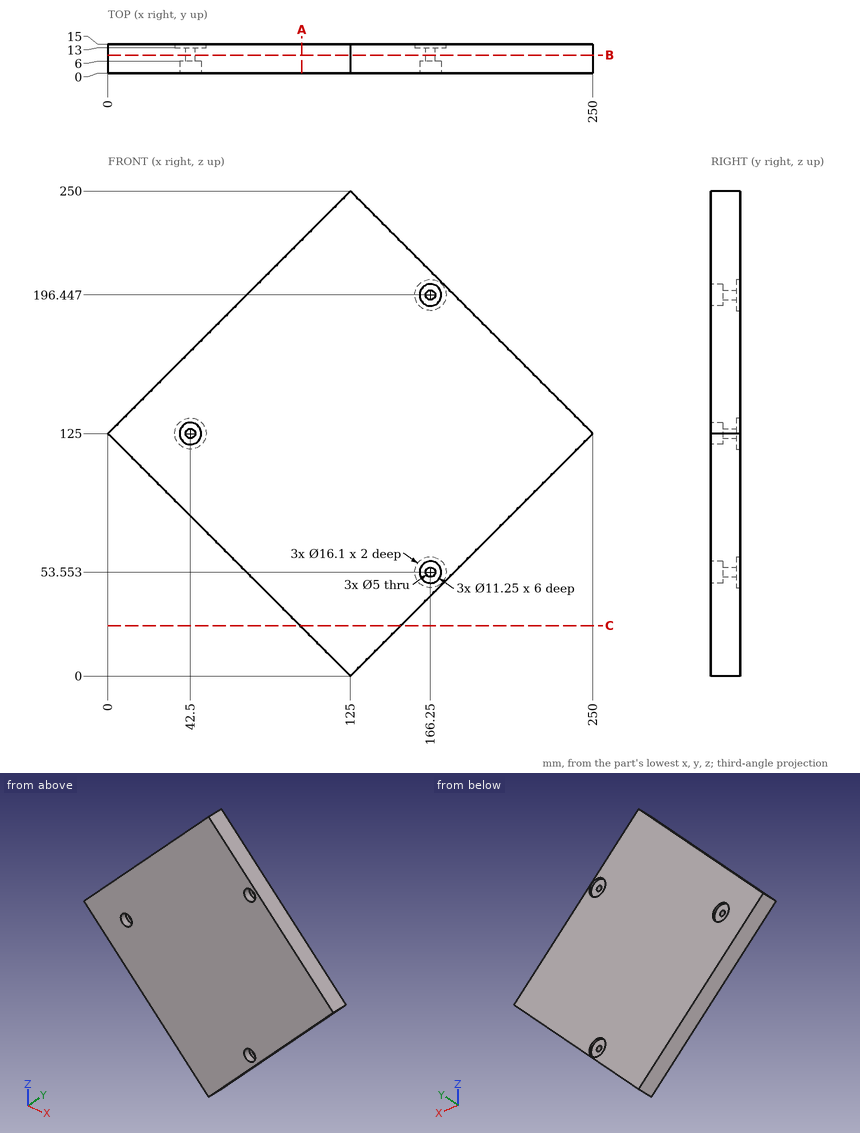
Here's the drawing with two shaded views (mm, measured from the low corner). I have some questions. Coordinates: 2 decimals unless noted, no trailing zeros. Write each loop counter-clockwise with the first axis right and the second up, starting at its lowest first coordinate (ties: lowest second). Pieces come first, ordered by that corner, then holes. Notation, with made-up numbers: (18.5, -24) -> (22.5, -24) arc R28 ccw to (22.5, 4) -> close; hole circle Ø1 at (45.5, 5). An arc over 180 degrees is marked (long way). Write item = value, one per line. Start each with the question number.
(1) Will these pins go through, and if not, where does the flat tip stop? pin 1 (4 mm diameter, centred on x = 93.5, y = 2.5, fed in from +Z); pin 2 (3.5 mm diameter, centred on x = 168.5, z = 53.5, fed in from -Y); pin 3 (1.5 mm diameter, centred on y = 10, z = 132, fed in from +X).
(2) I want a section at C-C (z = 26). Please give me the cut outline in (x, y).
(3) I want a section at A-A (x = 100). Please give me the cut outline in (y, z), plus the area to 3 significant figures.
(4) I need wall thicknesses on line 1 (Z direction, x = 166.25, y = 14.35); line 2 (Z direction, x = 42.5, y = 8.5); line 3 (Z direction, x = 15.5, y = 3.5). Which ranges of each line are inside material? Lowest first, please. Write a range as [from, to].
(5) I want a section at B-B (y = 9.25). Please give me the cut outline in (x, z), plus the area to 3 significant figures.
Result set:
q1.pin_1 = 220.5
q1.pin_2 = 6
q1.pin_3 = 243.75
q2.outline = (99, 0) -> (151, 0) -> (151, 15) -> (99, 15) -> close
q3.outline = (0, 25) -> (15, 25) -> (15, 225) -> (0, 225) -> close
q3.area = 3,000 mm2
q4.line_1 = [41.25, 45.5], [61.6, 188.4], [204.5, 208.75]
q4.line_2 = [82.5, 122.5], [127.5, 167.5]
q4.line_3 = [109.5, 140.5]
q5.outline = (0, 125) -> (125, 0) -> (250, 125) -> (125, 250) -> close; hole circle Ø5 at (42.5, 125); hole circle Ø5 at (166.25, 53.55); hole circle Ø5 at (166.25, 196.45)
q5.area = 31,200 mm2
